from build123d import *

# Parameters (mm, degrees)
F1_DEPTH = 9.525
F2_R     = 9.525
F3_DEPTH = 1.5875


with BuildPart() as f1:
    # F0 (on Front) → F1 (new body)
    with BuildSketch(Plane.XZ):
        with BuildLine():
            Line((42.493247, -88.9), (8.950572, 3.257742))
            ThreePointArc((8.950572, 3.257742), (0, 9.525), (-8.950572, 3.257742))
            Line((-8.950572, 3.257742), (-42.493247, -88.9))
            Line((-42.493247, -88.9), (0, -88.9))
            Line((0, -88.9), (42.493247, -88.9))
        make_face()
    extrude(amount=F1_DEPTH)

    # F2 (on face) → F3 (join)
    with BuildSketch(Plane.XZ.offset(9.525)):
        Circle(F2_R)
    extrude(amount=F3_DEPTH)


solid = f1.part
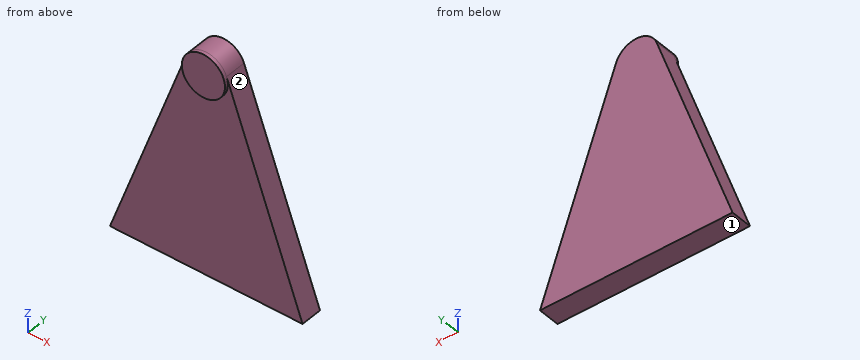
Read the model definition and answer for the solid it produces. Units are mm, in the model's axes. Face numbers are marked on the shaded views. Give positions to 0.01 mm unless a question says otherwise; leave off trailing zeros. Write each loop counter-clockwise with the first axis right and the second up, starting at its lowest first coordinate (ties: lowest second). Pieces come first, ordered by that corner, then holes. Notation, with made-up numbers: (58, 71.25) - (83, 71.25) arc R24 ccw to (83, 81.25) - close; hole circle Ø5 at (-5, 30). An arc over 180 degrees is marked (long way). Return JSON: item names as keys, results as strings.
Q1. Consider line 1 along Y through (x, z) = (17.5, -45) (3 decimals); line 2 along X through (y, z) = (-10.25, -0.5); line 3 along X through (y, z) = (-8, -63). Determine where each line is inside the solid, lowest interval first. Write a range as [from, to].
Reply:
{"line 1": "[-9.525, 0]", "line 2": "[-9.51, 9.51]", "line 3": "[-33.07, 33.07]"}
Q2. A cutting plane is placed at A-A, the plane z = 0. Determine the outline of the cut face in (x, y) (1 decimal).
Reply:
{"outline": "(-10.1, -9.5) - (-9.5, -9.5) - (-9.5, -11.1) - (9.5, -11.1) - (9.5, -9.5) - (10.1, -9.5) - (10.1, 0) - (-10.1, 0) - close"}
Q3. A cutting plane is placed at D-D, the plane x = 30.5. Determine the outline of the cut face in (y, z) (3 decimals).
Reply:
{"outline": "(-9.525, -88.9) - (0, -88.9) - (0, -55.949) - (-9.525, -55.949) - close"}
Q4. For a pull along X with two mould halves and no side action, classify the marked faces 1 and 2 as released by +X, released by -X, zero draft, split by the parting line, or undercut.
Reply:
{"face 1": "zero draft", "face 2": "released by +X"}
Q5. A cutting plane is placed at B-B, the plane x = 0. Determine the outline of the cut face in (y, z) (1 decimal), and give its area (3 significant figures).
Reply:
{"outline": "(-11.1, -9.5) - (-9.5, -9.5) - (-9.5, -88.9) - (0, -88.9) - (0, 9.5) - (-11.1, 9.5) - close", "area": "968 mm²"}
Q6. Given P1, Ø6, axis at x = 4, z = -31, coming from the -Y side (3 decimals); P2, Ø10, axis at x = -12, z = -62.5, coming from the +Y side; P3, Ø4, axis at y = -7.5, z = -37, coming from the -X side; P4, Ø3, axis at y = -7.5, z = -50.5, coming from the -X side, each flat-ended and moving along its own axis, determine where each tip first touches the part or whether it passes through.
Reply:
{"P1": "y = -9.525", "P2": "y = 0", "P3": "x = -24.33", "P4": "x = -29.06"}
Q7. A cutting plane is placed at C-C, the plane y = -6. Determine the outline of the cut face in (x, z) (3 decimals).
Reply:
{"outline": "(-42.493, -88.9) - (42.493, -88.9) - (8.951, 3.258) arc R9.525 ccw to (-8.951, 3.258) - close"}
